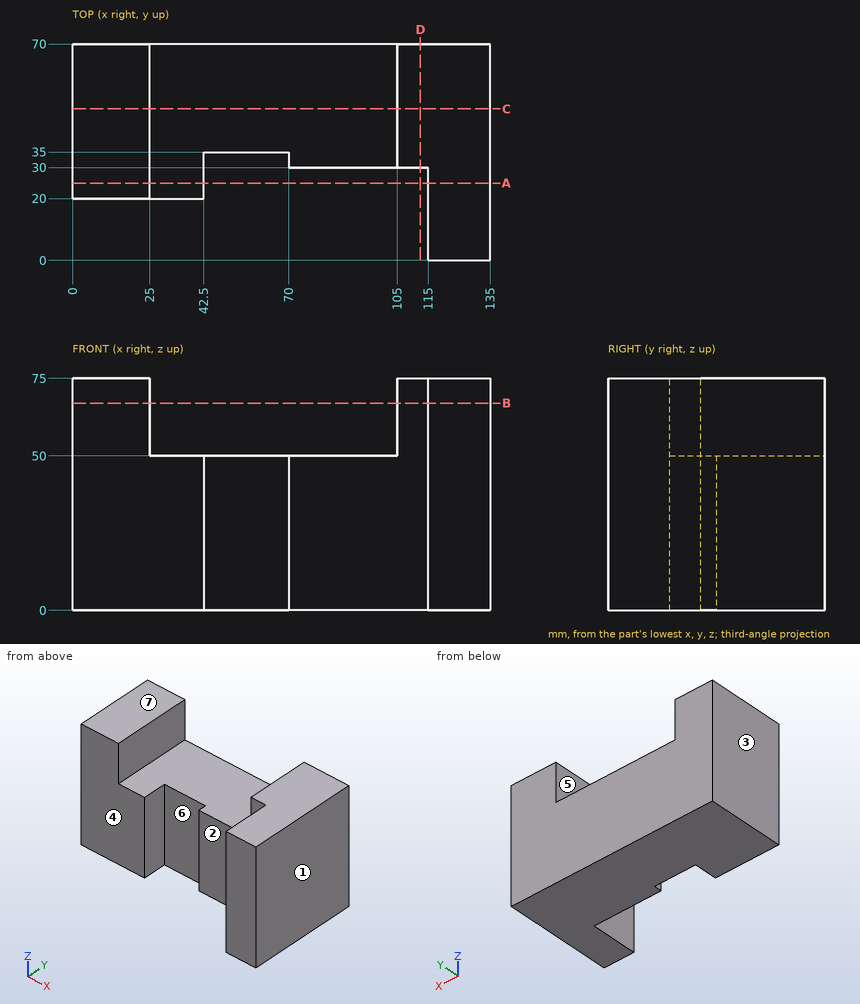
Geometry check sheet. Reference: drawing and pictorial views, mm from the part's lowest x, y, z. A direction names the side the tool comes from. Coordinates: 2 decimals unless noted, no trailing zeros. Write each loop counter-clockwise with the first axis right and the second up, starting at its lowest first coordinate (ties: lowest second). Pieces come first, ordered by that corner, then holes. Notation, with made-up numbers: (-11, -2.5) - (0, -2.5) arc R7 cw to (0, 5.5) - close; hole circle Ø1 at (4.25, -2). An arc over 180 degrees is marked (long way). One line per question, with ' | ' between items. Start each with the question number.
1. Draft check along X on the marked faces 1, 2, 3 and 4. Enter one of: released by +X, released by -X, zero draft, split by the parting line, or undercut.
2. Section check B-B (z = 67). Enter the section's corners in (x, y).
3. Access from +Z, -Z, +X, -X, +Y, -Y to the whole of each face (thin tool, end or side, straight path). Record for the marked faces 5, 6 and 7.
4. Section check A-A (y = 25). Enter the section's corners in (x, z), plus the area to 3 significant figures.
5. Material ranges on line 1 along X through (y, z) = (22, 23); line 2 along X through (y, z) = (31, 70.5); line 3 along Y through (x, z) = (104, 25), recorded low to high.
6. Gauge pin test, flat ends, axial feed: P1, Ø5, axis at x = 58.5, z = 14, coming from the -Y side; P2, Ø2, axis at x = 84, y = 40.5, coming from the +Z side; P3, Ø13, axis at x = 20.5, z = 22, coming from the -Y side. Record the tip position at first contact, or that the pin passes through.
7. Section check C-C (y = 49). Enter the section's corners in (x, z).
8. Section check D-D (x = 112.5). Enter the section's corners in (y, z).
Computed values:
1) face 1: released by +X | face 2: undercut | face 3: released by -X | face 4: zero draft
2) outline: (0, 20) - (25, 20) - (25, 70) - (0, 70) - close; (105, 30) - (115, 30) - (115, 0) - (135, 0) - (135, 70) - (105, 70) - close
3) face 5: +Z, +Y, -Y | face 6: +Z, -Z, -Y | face 7: +Z, +X, -X, +Y, -Y
4) outline: (0, 0) - (42.5, 0) - (42.5, 50) - (25, 50) - (25, 75) - (0, 75) - close; (115, 0) - (135, 0) - (135, 75) - (115, 75) - close | area: 4,250 mm²
5) line 1: 0 to 42.5, 115 to 135 | line 2: 0 to 25, 105 to 135 | line 3: 30 to 70
6) P1: y = 35 | P2: z = 50 | P3: y = 20
7) outline: (0, 0) - (135, 0) - (135, 75) - (105, 75) - (105, 50) - (25, 50) - (25, 75) - (0, 75) - close
8) outline: (30, 0) - (70, 0) - (70, 75) - (30, 75) - close
